Check sheet for the modelled part. Datum: model origin and axes. Units: mm. A direction names the side the tool comes from. Coordinates: 2 decimals unless noted, no trailing zeros. Write each question's results on one line, items separated by ' | '. Start each with the question number.
from build123d import *

# Parameters (mm, degrees)
F1_FACE_R       = 7.62
F5_DEPTH        = 25.4
F5_COPIES_COUNT = 10


# Not quite as in the source:
# - a pattern or mirror of a feature is missing from the dataset's text; its kind, count and spacing are read off the source's solid


with BuildPart() as f1:
    # F0 (on Front) → F1 (revolve)
    with BuildSketch(Plane.XZ):
        with BuildLine():
            Line((-7.62, 4.3819724477), (-7.62, -5.1430275523))
            Line((-7.62, -5.1430275523), (0, -5.1430275523))
            Line((0, -5.1430275523), (0, 12.0019724477))
            ThreePointArc((0, 12.0019724477), (-5.3881536726, 9.7701261203), (-7.62, 4.3819724477))
        make_face()
    revolve(axis=Axis((0, 0, 3.4294724477), (0, 0, -1)))

    # F1_face (on face) → F2 section 0
    with BuildSketch(Plane(origin=(0, 0, -5.1430275523), x_dir=(1, 0, 0), z_dir=(0, 0, -1)), mode=Mode.PRIVATE) as f2_s0:
        Circle(F1_FACE_R)
    loft([f2_s0.sketch, Vertex(0, 0, 0)], mode=Mode.SUBTRACT)

    # F4 (on offset) → F5 (cut)
    with BuildSketch(Plane.XZ.offset(5.08)):
        Polygon((6.7222419615, -10.7367794649), (7.8839848078, -10.2236970553), (-11.1258903258, 32.8192645344), (-12.2876331722, 32.3061821249), align=None)
    f5 = extrude(amount=F5_DEPTH, mode=Mode.SUBTRACT)

    # F5_copies: F5 ×10 about axis
    f5_copies_axis = Axis((0, 0, 0), (0, 0, 1))
    for i in range(1, F5_COPIES_COUNT):
        add(f5.rotate(f5_copies_axis, i * 360 / F5_COPIES_COUNT), mode=Mode.SUBTRACT)


solid = f1.part
1) Set-up check for faces 4 (the flat face through (-5.215, -3.386, 3.985)), 5 (the flat face through (-2, 5.08, 2)), 6 (the flat face through (4.326, -4.335, 2.329)): record each of +Z, -Z, +X, -X, +Y, -Y from which the full face is reachable in a straight line by a thin tool's end or side.
2) Release check for a two-part mould opening along Y. For faces 1 (the cylindrical face through (-4.98, 5.77, -0.45)), 2 (the flat face through (-1.64, -5.09, 2.46)), 3 (the cylindrical face through (4.98, -5.77, -0.45)) record: +Y half, -Y half, draft (parallel to the pull), parting line (faces both ways), or undercut.
3) Thickness scan on probe 1 along X at (y, z) = (-1.25, -4); probe 2 along X at (y, z) = (-4.5, 4.75); probe 3 along Y at (x, z) = (-2.75, -3.75). Record the ranges inside material, lowest first.
4) Gauge pin test, flat ends, axial feed: P1, Ø8, axis at y = 4.5, z = 3.5, coming from the -X side; P2, Ø5, axis at y = -4, z = 3.5, coming from the -X side; P3, Ø3, axis at x = 1, y = 5.5, coming from the +Z side. Record the tip position at first contact, or that the pin passes through.
Return value:
1) face 4: -X | face 5: +Y | face 6: none
2) face 1: +Y half | face 2: undercut | face 3: -Y half
3) probe 1: x = -7.52 to -5.79, 5.79 to 6.92, 7.26 to 7.52 | probe 2: x = -6.14 to -3.41, -2.45 to 3.12, 4.84 to 6.14 | probe 3: y = -7.11 to -4.83, 4.83 to 7.11
4) P1: stops at x = -7.6 | P2: stops at x = -7.47 | P3: stops at z = 10.81
